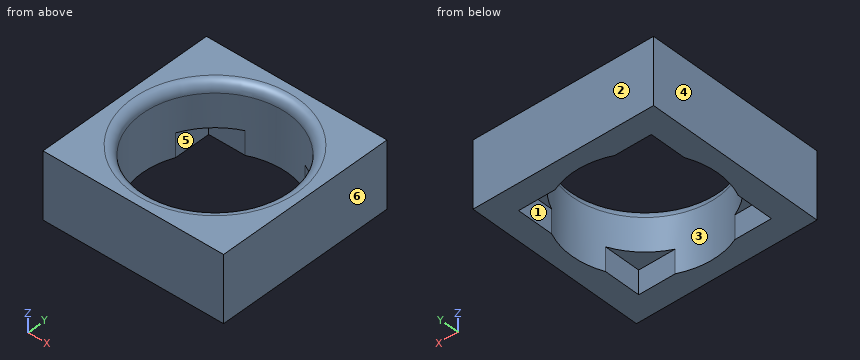
Autodesk Fusion 360 part; units mm, degrees
sketch "Sketch1" plane through (0, 0, 0) normal (0, 0, 1) x (1, 0, 0)
  line L0 (0, 0) -> (19.05, 0)
  line L1 (19.05, 0) -> (19.05, 19.05)
  line L2 (19.05, 19.05) -> (0, 19.05)
  line L3 (0, 19.05) -> (0, 0)
  line L4 (0, 0) -> (19.05, 19.05) construction
  line L5 (0, 19.05) -> (19.05, 0) construction
  circle A0 centre (9.525, 9.525) radius 7.675
  line L6 (16.525, 2.525) -> (2.525, 2.525)
  line L7 (2.525, 2.525) -> (2.525, 16.525)
  line L8 (2.525, 16.525) -> (16.525, 16.525)
  line L9 (16.525, 16.525) -> (16.525, 2.525)
  line L10 (16.525, 2.525) -> (2.525, 16.525) construction
  line L11 (2.525, 2.525) -> (16.525, 16.525) construction
  point P0 (9.525, 9.525)
  dimension "d1" = 19.05
  dimension "d2" = 19.05
  dimension "d5" = 15.35
  dimension "d6" = 14
  dimension "d7" = 14
extrude "Extrude1" add sketch "Sketch1" along normal blind 7 contours L0 L1 L2 L3 | A0 L8 L9 | A0 L6 L9 | A0 L7 L8 | A0 L6 L7
extrude "Extrude2" cut sketch "Sketch1" along normal blind 2.5 contours A0 L8 L9 | A0 L6 L9 | A0 L7 L8 | A0 L6 L7
fillet "Fillet1" radius 1 1 edges at (2.3694, 12.3004, 7)
equation "d1 = width"
equation "d2 = height"
equation "encoder_diameter = 15.35 mm"
equation "encoder_cutout = 14 mm"
equation "d5 = encoder_diameter"
equation "d6 = encoder_cutout"
equation "d7 = encoder_cutout"
equation "shell_thickness = 7 mm"
equation "encoder_cut_height = 2.5 mm"
equation "d10 = shell_thickness"
equation "d12 = encoder_cut_height"
equation "height = 19.05 mm"
equation "width = 19.05 mm"
For this review, take the finished solid that the model builds, in its own axes (mm). Face numbers are marked on the shaded views. A direction names the side the tool comes from. Coordinates: 2 decimals unless noted, no trailing zeros. Loops run counter-clockwise (first coordinate to the right, second up) from the corner with the lowest first, then second, coordinate; pieces in that order, holes last. Notation, with made-up numbers: (34.25, 24.5) - (41.25, 24.5) arc R17 ccw to (41.25, 54.5) - close; hole circle Ø8 at (86, -17.75). An arc over 180 degrees is marked (long way). Use a Markdown table: item, result. Add a question column.
Item 1: Insertion check: pin 1 Ø1.2 at (x, y) = (14.5, 4) entering from -Z; pin 2 Ø9 at (x, y) = (9.525, 9.525) entering from -Z. Each pin has a flat end and moves straight along its axis. Give the tip position at first contact, or say it passes through.
Item 2: We need section A-A (z = 0.75). Give the boundary of the cut face in (x, y) (3 decimals), and give its area (3 significant figures).
Item 3: Mouldability with a two-part tool opening along Y and no side actions: class the marked faces 1, 2, 3 and 4 as pulls with the +Y half, pulls with the -Y half, needs draft (parallel to the pull), parting line crosses it, or undercut.
Item 4: For line 1 (Y direction, x = 3, z = 2) (3 decimals); line 2 (Y direction, x = 9.5, z = 5.25), list the stretches that pass through material, from the lowest coordinate up.
Item 5: Tool access review of the marked faces 5 and 6: name each direction out of +Z, -Z, +X, -X, +Y, -Y from which nothing blocks a thin tool from reaching the whole face with its end or side.
Item 6: We need section B-B (z = 2.75). Give the boundary of the cut face in (x, y) (3 decimals), and give its area (3 significant figures).
Results list:
| question | item | result |
|---|---|---|
| 1 | pin 1 | stops at z = 2.5 |
| 1 | pin 2 | passes through |
| 2 | outline | (0, 0) - (19.05, 0) - (19.05, 19.05) - (0, 19.05) - close; hole (2.525, 2.525) - (6.378, 2.525) arc R7.675 ccw to (12.672, 2.525) - (16.525, 2.525) - (16.525, 6.378) arc R7.675 ccw to (16.525, 12.672) - (16.525, 16.525) - (12.672, 16.525) arc R7.675 ccw to (6.378, 16.525) - (2.525, 16.525) - (2.525, 12.672) arc R7.675 ccw to (2.525, 6.378) - close |
| 2 | area | 155 mm^2 |
| 3 | face 1 | undercut |
| 3 | face 2 | pulls with the +Y half |
| 3 | face 3 | undercut |
| 3 | face 4 | needs draft |
| 4 | line 1 | y = 0 to 2.525, 16.525 to 19.05 |
| 4 | line 2 | y = 0 to 1.85, 17.2 to 19.05 |
| 5 | face 5 | -Z |
| 5 | face 6 | +Z, -Z, +X, +Y, -Y |
| 6 | outline | (0, 0) - (19.05, 0) - (19.05, 19.05) - (0, 19.05) - close; hole circle Ø15.35 at (9.525, 9.525) |
| 6 | area | 178 mm^2 |
